Could you check a few things on this model? Use its own coordinates, in mm. Give positions to 0.01 mm unless a question says otherwise; leave off trailing zeros. Write each question's results on one line, items separated by ' | '. Start each with the question number.
(1) I need wall thicknesses on line 1 (Y direction, x = -49.5, z = 0.85); line 2 (Y direction, x = -27.5, z = 0.7); line 3 (X direction, y = -28, z = 0.65). Which ranges of each line are inside material? Lowest first, please.
(2) Suppose I cut it at A-A (z = 1.25). Count the separate pieces of the cut face and the enclosed holes in it, and give its area (3 significant figures).
(3) For pin 1 (1.7 mm diameter, centred on x = 49.5, y = -27.5, fed in from +Z); pin 2 (0.8 mm diameter, centred on x = -45.5, z = 0.5, fed in from -Y); pin 3 (0.5 mm diameter, centred on x = 51, z = 1, fed in from -Y); pin 4 (0.8 mm diameter, centred on y = -47, z = 1, fed in from -X), each with a flat end and sliding along its axis, tell me the tip position at first contact or that it passes through.
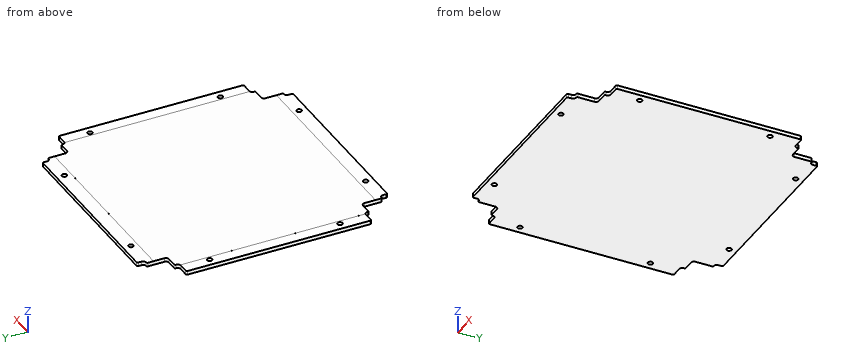
from build123d import *

# Parameters (mm, degrees)
SKETCH1_W                 = 106
SKETCH1_H                 = 106
MAINOUTLINE_DEPTH         = 1.6
SKETCH4_W                 = 11.7
SKETCH4_H                 = 11.7
RAILCUTOUTS_DEPTH         = 2.6
FILLETCUTOUTS_START       = -2.6
SKETCH13_W                = 5.7
SKETCH13_H                = 1.9
SKETCH13_W_2              = 1.8
SKETCH13_H_2              = 3
FILLETCUTOUTS_DEPTH       = 3.6
SMOOTHCORNER_DEPTH        = 10
MIRROR2_COPY_1_SKETCH_W   = 11.7
MIRROR2_COPY_1_SKETCH_H   = 11.7
MIRROR2_COPY_1_DEPTH      = 2.6
MIRROR2_START             = -2.6
MIRROR2_COPY_2_SKETCH_W   = 5.7
MIRROR2_COPY_2_SKETCH_H   = 1.9
MIRROR2_COPY_2_SKETCH_W_2 = 1.8
MIRROR2_COPY_2_SKETCH_H_2 = 3
MIRROR2_COPY_2_DEPTH      = 3.6
MIRROR2_COPY_3_DEPTH      = 10
MIRROR2_COPY_4_SKETCH_W   = 11.7
MIRROR2_COPY_4_SKETCH_H   = 11.7
MIRROR2_COPY_4_DEPTH      = 2.6
MIRROR2_COPY_5_SKETCH_W   = 5.7
MIRROR2_COPY_5_SKETCH_H   = 1.9
MIRROR2_COPY_5_SKETCH_W_2 = 1.8
MIRROR2_COPY_5_SKETCH_H_2 = 3
MIRROR2_COPY_5_DEPTH      = 3.6
FILLET10_R                = 0.5
M2_CLEARANCE_HOLE1_D      = 2.1
SKETCH16_W                = 90
SKETCH16_H                = 6.2
SKETCH16_W_2              = 5.2
SKETCH16_H_2              = 90
CUT_EXTRUDE6_DEPTH        = 0.001
SKETCH24_OUTSIDE_W        = 137.984
SKETCH24_OUTSIDE_H        = 137.984
SKETCH24_OUTSIDE_W_2      = 105.6
SKETCH24_OUTSIDE_H_2      = 105.6
CUT_EXTRUDE19_DEPTH       = 2.6
FILLET7_R                 = 0.5


with BuildPart() as part:
    # Sketch1 → mainOutline (new body)
    with BuildSketch(Plane.XY):
        Rectangle(SKETCH1_W, SKETCH1_H)
    extrude(amount=MAINOUTLINE_DEPTH)

    # Sketch4 → railCutouts (cut, through all)
    with BuildSketch(Plane(origin=(0, 0, 0), x_dir=(-1, 0, 0), z_dir=(0, 0, -1))):
        with Locations((47.15, 47.15)):
            Rectangle(SKETCH4_W, SKETCH4_H)
    railcutouts = extrude(amount=-RAILCUTOUTS_DEPTH, mode=Mode.SUBTRACT)

    # Sketch13 → filletCutouts (cut)
    with BuildSketch(Plane(origin=(0, 0, 0), x_dir=(-1, 0, 0), z_dir=(0, 0, -1)).offset(FILLETCUTOUTS_START)):
        with Locations((50.15, 40.35)):
            Rectangle(SKETCH13_W, SKETCH13_H)
        with Locations((40.4, 51.5)):
            Rectangle(SKETCH13_W_2, SKETCH13_H_2)
    filletcutouts = extrude(amount=FILLETCUTOUTS_DEPTH, mode=Mode.SUBTRACT)

    # Sketch27 → smoothCorner (cut)
    with BuildSketch(Plane.XY.offset(1.6)):
        with BuildLine():
            Line((-40.928025612, 42.198025612), (-40.928025612, 49.628025612))
            Line((-40.928025612, 49.628025612), (-40.398025612, 49.628025612))
            ThreePointArc((-40.398025612, 49.628025612), (-39.5, 50), (-39.128025612, 50.898025612))
            Line((-39.128025612, 50.898025612), (-39.128025612, 53))
            Line((-39.128025612, 53), (-53, 53))
            Line((-53, 53), (-53, 39.028025612))
            Line((-53, 39.028025612), (-48.198025612, 39.028025612))
            ThreePointArc((-48.198025612, 39.028025612), (-47.3, 39.4), (-46.928025612, 40.298025612))
            Line((-46.928025612, 40.298025612), (-46.928025612, 40.928025612))
            Line((-46.928025612, 40.928025612), (-42.198025612, 40.928025612))
            ThreePointArc((-42.198025612, 40.928025612), (-41.3, 41.3), (-40.928025612, 42.198025612))
        make_face()
    smoothcorner = extrude(amount=-SMOOTHCORNER_DEPTH, mode=Mode.SUBTRACT)

    # Mirror1: railCutouts, filletCutouts, smoothCorner across plane
    add(railcutouts.mirror(Plane(origin=(0, 0, 0), x_dir=(0, 0, 1), z_dir=(1, 0, 0))), mode=Mode.SUBTRACT)
    add(filletcutouts.mirror(Plane(origin=(0, 0, 0), x_dir=(0, 0, 1), z_dir=(1, 0, 0))), mode=Mode.SUBTRACT)
    add(smoothcorner.mirror(Plane(origin=(0, 0, 0), x_dir=(0, 0, 1), z_dir=(1, 0, 0))), mode=Mode.SUBTRACT)

    # Mirror2: smoothCorner across plane
    add(smoothcorner.mirror(Plane.ZX), mode=Mode.SUBTRACT)

    # Mirror2 copy 1 sketch → Mirror2 copy 1 (cut, through all)
    with BuildSketch(Plane(origin=(0, 0, 0), x_dir=(1, 0, 0), z_dir=(0, 0, -1))):
        with Locations((47.15, 47.15)):
            Rectangle(MIRROR2_COPY_1_SKETCH_W, MIRROR2_COPY_1_SKETCH_H)
    extrude(amount=-MIRROR2_COPY_1_DEPTH, mode=Mode.SUBTRACT)

    # Mirror2 copy 2 sketch → Mirror2 copy 2 (cut)
    with BuildSketch(Plane(origin=(0, 0, 0), x_dir=(1, 0, 0), z_dir=(0, 0, -1)).offset(MIRROR2_START)):
        with Locations((50.15, 40.35)):
            Rectangle(MIRROR2_COPY_2_SKETCH_W, MIRROR2_COPY_2_SKETCH_H)
        with Locations((40.4, 51.5)):
            Rectangle(MIRROR2_COPY_2_SKETCH_W_2, MIRROR2_COPY_2_SKETCH_H_2)
    extrude(amount=MIRROR2_COPY_2_DEPTH, mode=Mode.SUBTRACT)

    # Mirror2 copy 3 sketch → Mirror2 copy 3 (cut)
    with BuildSketch(Plane(origin=(0, 0, 1.6), x_dir=(-1, 0, 0), z_dir=(0, 0, 1))):
        with BuildLine():
            Line((-40.928025612, 42.198025612), (-40.928025612, 49.628025612))
            Line((-40.928025612, 49.628025612), (-40.398025612, 49.628025612))
            ThreePointArc((-40.398025612, 49.628025612), (-39.5, 50), (-39.128025612, 50.898025612))
            Line((-39.128025612, 50.898025612), (-39.128025612, 53))
            Line((-39.128025612, 53), (-53, 53))
            Line((-53, 53), (-53, 39.028025612))
            Line((-53, 39.028025612), (-48.198025612, 39.028025612))
            ThreePointArc((-48.198025612, 39.028025612), (-47.3, 39.4), (-46.928025612, 40.298025612))
            Line((-46.928025612, 40.298025612), (-46.928025612, 40.928025612))
            Line((-46.928025612, 40.928025612), (-42.198025612, 40.928025612))
            ThreePointArc((-42.198025612, 40.928025612), (-41.3, 41.3), (-40.928025612, 42.198025612))
        make_face()
    extrude(amount=-MIRROR2_COPY_3_DEPTH, mode=Mode.SUBTRACT)

    # Mirror2 copy 4 sketch → Mirror2 copy 4 (cut, through all)
    with BuildSketch(Plane(origin=(0, 0, 0), x_dir=(-1, 0, 0), z_dir=(0, 0, -1))):
        with Locations((47.15, -47.15)):
            Rectangle(MIRROR2_COPY_4_SKETCH_W, MIRROR2_COPY_4_SKETCH_H)
    extrude(amount=-MIRROR2_COPY_4_DEPTH, mode=Mode.SUBTRACT)

    # Mirror2 copy 5 sketch → Mirror2 copy 5 (cut)
    with BuildSketch(Plane(origin=(0, 0, 0), x_dir=(-1, 0, 0), z_dir=(0, 0, -1)).offset(MIRROR2_START)):
        with Locations((50.15, -40.35)):
            Rectangle(MIRROR2_COPY_5_SKETCH_W, MIRROR2_COPY_5_SKETCH_H)
        with Locations((40.4, -51.5)):
            Rectangle(MIRROR2_COPY_5_SKETCH_W_2, MIRROR2_COPY_5_SKETCH_H_2)
    extrude(amount=MIRROR2_COPY_5_DEPTH, mode=Mode.SUBTRACT)

    # Fillet10
    fillet10_edges = [part.edges().sort_by_distance(p)[0] for p in [
        (40.928025612, 49.628025612, 0.8),
        (46.928025612, 40.928025612, 0.8),
        (46.928025612, -40.928025612, 0.8),
        (40.928025612, -49.628025612, 0.8),
        (-40.928025612, -49.628025612, 0.8),
        (-46.928025612, -40.928025612, 0.8),
        (-46.928025612, 40.928025612, 0.8),
        (-40.928025612, 49.628025612, 0.8),
    ]]
    fillet(fillet10_edges, radius=FILLET10_R)

    # M2 Clearance Hole1 (through all)
    with Locations(Plane(origin=(0, 0, 0), x_dir=(-1, 0, 0), z_dir=(0, 0, -1))):
        with Locations((49.5, -27.5), (27.5, -49.5), (-49.5, -27.5), (-27.5, -49.5), (-27.5, 49.5), (-49.5, 27.5), (27.5, 49.5), (49.5, 27.5)):
            Hole(M2_CLEARANCE_HOLE1_D / 2)

    # Sketch16 → Cut-Extrude6 (cut)
    with BuildSketch(Plane.XY.offset(1.6)):
        with Locations((0, -49.9)):
            Rectangle(SKETCH16_W, SKETCH16_H)
        with Locations((0, 49.9)):
            Rectangle(SKETCH16_W, SKETCH16_H)
        with Locations((-50.4, 0)):
            Rectangle(SKETCH16_W_2, SKETCH16_H_2)
        with Locations((50.4, 0)):
            Rectangle(SKETCH16_W_2, SKETCH16_H_2)
    extrude(amount=-CUT_EXTRUDE6_DEPTH, mode=Mode.SUBTRACT)

    # Sketch24 outside → Cut-Extrude19 (cut, through all)
    with BuildSketch(Plane.XY.offset(1.6)):
        Rectangle(SKETCH24_OUTSIDE_W, SKETCH24_OUTSIDE_H)
        Rectangle(SKETCH24_OUTSIDE_W_2, SKETCH24_OUTSIDE_H_2, mode=Mode.SUBTRACT)
    extrude(amount=-CUT_EXTRUDE19_DEPTH, mode=Mode.SUBTRACT)

    # Fillet7
    fillet7_edges = [part.edges().sort_by_distance(p)[0] for p in [
        (-52.8, -39.028025612, 0.7995),
        (-39.128025612, -52.8, 0.7995),
        (52.8, -39.028025612, 0.7995),
        (39.128025612, 52.8, 0.7995),
        (52.8, 39.028025612, 0.7995),
        (39.128025612, -52.8, 0.7995),
        (-52.8, 39.028025612, 0.7995),
        (-39.128025612, 52.8, 0.7995),
    ]]
    fillet(fillet7_edges, radius=FILLET7_R)


solid = part.part
Output values:
1) line 1: -39.03 to -28.55, -26.45 to 26.45, 28.55 to 39.03 | line 2: -52.8 to -50.55, -48.45 to 48.45, 50.55 to 52.8 | line 3: -52.8 to -50.42, -48.58 to 48.58, 50.42 to 52.8
2) separate pieces: 1 | enclosed holes: 8 | area: 10,500 mm2
3) pin 1: through | pin 2: y = -40.93 | pin 3: y = -39.03 | pin 4: x = -40.93
